Geometry: final body of the model. Coordinates: model frame, mm. A direction names the side the tool comes from. Round coordinates to 2 decimals unless told otherwise and drop trailing zeros. Loops run counter-clockwise (first coordinate to the right, second up) from the corner with the lowest first, then second, coordinate; pieces in that order, holes last. Notation, with made-up numbers: (74, 71.5) - (121, 71.5) arc R25 cw to (121, 108.5) - close; hole circle Ø11 at (17, 57). An arc over 180 degrees is marked (long way). Write item = value, one per line. Start each with the question number.
Item 1: Access query for faces 1 (the flat face through (-11, 33, -6.4)), 2 (the flat face through (-14.8, 74.2, -5.1)), 3 (the flat face through (-19.7, 74, -18)), 4 (the flat face through (-35, 74, -23.025)). Directions: +Z, -Z, +X, -X, +Y, -Y. A direction counts if a zero-diameter tool reaches every point of the face in a straight line with its end or side. Return the directions, or none.
Item 2: Section B-B (x = -32.7). Return loops of the section in (y, z) (3 decimals), plus the area to 3 significant figures.
Item 3: Section C-C (y = 71.5). Return loops of the section in (x, z) (3 decimals), plus the area to 3 significant figures.
Item 4: Draft query along Y for faces 5 (the flat face through (-45.7, 74, -18)), 6 (the cylindrical face through (-53.24, 50.96, 1.48)), 7 (the flat face through (-30, 85.4, -2)). Return one class per face: pulls with the +Y half, pulls with the -Y half, needs draft (parallel to the pull), parting line crosses it, or undercut.
Item 5: Line query: line 1 (Y direction, x = -12.7, z = 0.9); line 2 (Z direction, x = -37, y = 67) (3 decimals); line 3 (Y direction, x = -32.7, z = -25.2). Output: solid intervals per line, ascending. Write a range as from..to.
Item 6: Section D-D (y = 32.7). Return loops of the section in (x, z).
Item 7: First-contact query: pin 1 (1.2 mm diameter, centred on x = -55.5, y = 33, fed in from -Z); pin 2 (2 mm diameter, centred on x = -56, z = -7.5, fed in from +Y); pin 3 (6 mm diameter, centred on y = 74, z = -13.5, fed in from -X); pin 4 (4 mm diameter, centred on x = -24.5, z = -16.5, fed in from +Y). Flat tips, straight axial feed; report the tip coordinate or a pass-through.
Item 8: Section A-A (y = 12). Return loops of the section in (x, z), plus the area to 3 significant figures.
from build123d import *

# Parameters (mm, degrees)
SKETCH_1_W             = 65.4
SKETCH_1_H             = 85.4
SKETCH_1_R             = 2.5
EXTRUDE_632_DEPTH      = 3
SKETCH_2_W             = 26
SKETCH_2_H             = 22
EXTRUDE_871_DEPTH      = 26
SKETCH_3_W             = 20.05
SKETCH_3_H             = 20.05
CUT_EXTRUDE_1082_DEPTH = 95.724442463
SKETCH_8_R             = 5.872551453
EXTRUDE_1_DEPTH        = 14.4
SKETCH_4_R             = 2
EXTRUDE_3_DEPTH        = 14.4
SKETCH_12_R            = 5
EXTRUDE_5_DEPTH        = 21
SKETCH_13_R            = 2
CUT_EXTRUDE_1_DEPTH    = 6.6
SKETCH_14_R            = 2
CUT_EXTRUDE_3_DEPTH    = 8
CHAMFER_1_SIZE         = 10
CHAMFER_2_SIZE         = 10
SKETCH_15_R            = 2
CUT_EXTRUDE_4_DEPTH    = 8


with BuildPart() as part:
    # Эскиз1 → Extrude 632 (new body)
    with BuildSketch(Plane.XY):
        with Locations((-32.7, 42.7)):
            Rectangle(SKETCH_1_W, SKETCH_1_H)
        with Locations((-52.7, 53.4)):
            Circle(SKETCH_1_R, mode=Mode.SUBTRACT)
        with Locations(Location((-12.7, 53.4, 0), (0, 0, 180))):
            Circle(SKETCH_1_R, mode=Mode.SUBTRACT)
        with Locations((-12.7, 12)):
            Circle(SKETCH_1_R, mode=Mode.SUBTRACT)
        with Locations(Location((-52.7, 12, 0), (0, 0, 180))):
            Circle(SKETCH_1_R, mode=Mode.SUBTRACT)
    extrude(amount=EXTRUDE_632_DEPTH)

    # Эскиз2 → Extrude 871 (add)
    with BuildSketch(Plane(origin=(0, 0, 0), x_dir=(-1, 0, 0), z_dir=(0, 0, -1))):
        with Locations((32.7, 74.4)):
            Rectangle(SKETCH_2_W, SKETCH_2_H)
    extrude(amount=EXTRUDE_871_DEPTH)

    # Эскиз3 → Cut-Extrude 1082 (cut, through all)
    with BuildSketch(Plane.XZ.offset(-63.4)):
        with Locations((-32.7, -13)):
            Rectangle(SKETCH_3_W, SKETCH_3_H)
    extrude(amount=-CUT_EXTRUDE_1082_DEPTH, mode=Mode.SUBTRACT)

    # Эскиз8 → Бобышка-Вытянуть1 (add)
    with BuildSketch(Plane(origin=(0, 0, 0), x_dir=(-1, 0, 0), z_dir=(0, 0, -1))):
        with Locations(Location((10.7, 32.7, 0), (0, 0, 180))):
            Circle(SKETCH_8_R)
    extrude(amount=EXTRUDE_1_DEPTH)

    # Эскиз4 → Бобышка-Вытянуть3 (add)
    with BuildSketch(Plane(origin=(0, 0, 0), x_dir=(-1, 0, 0), z_dir=(0, 0, -1))):
        with Locations(Location((52.7, 32.7, 0), (0, 0, 180))):
            Circle(SKETCH_4_R)
    extrude(amount=EXTRUDE_3_DEPTH)

    # Эскиз12 → Бобышка-Вытянуть5 (add)
    with BuildSketch(Plane(origin=(0, 0, 0), x_dir=(-1, 0, 0), z_dir=(0, 0, -1))):
        with Locations(Location((54.7, 32.7, 0), (0, 0, 180))):
            Circle(SKETCH_12_R)
    extrude(amount=EXTRUDE_5_DEPTH)

    # Эскиз13 → Вырез-Вытянуть1 (cut)
    with BuildSketch(Plane(origin=(0, 0, -21), x_dir=(-1, 0, 0), z_dir=(0, 0, -1))):
        with Locations((54.7, 32.7)):
            Circle(SKETCH_13_R)
    extrude(amount=-CUT_EXTRUDE_1_DEPTH, mode=Mode.SUBTRACT)

    # Эскиз14 → Вырез-Вытянуть3 (cut)
    with BuildSketch(Plane(origin=(0, 0, -14.4), x_dir=(-1, 0, 0), z_dir=(0, 0, -1))):
        with Locations((10.7, 32.7)):
            Circle(SKETCH_14_R)
    extrude(amount=-CUT_EXTRUDE_3_DEPTH, mode=Mode.SUBTRACT)

    # Фаска1
    chamfer_1_edges = [part.edges().sort_by_distance(p)[0] for p in [
        (-45.7, 74.4, 0),
    ]]
    chamfer(chamfer_1_edges, length=CHAMFER_1_SIZE)

    # Фаска2
    chamfer_2_edges = [part.edges().sort_by_distance(p)[0] for p in [
        (-19.7, 74.4, 0),
    ]]
    chamfer(chamfer_2_edges, length=CHAMFER_2_SIZE)

    # Эскиз15 → Вырез-Вытянуть4 (cut)
    with BuildSketch(Plane(origin=(0, 0, -26), x_dir=(-1, 0, 0), z_dir=(0, 0, -1))):
        with Locations((32.7, 74.4)):
            Circle(SKETCH_15_R)
    extrude(amount=-CUT_EXTRUDE_4_DEPTH, mode=Mode.SUBTRACT)


solid = part.part
Taken from the geometry:
q1.face_1 = -Z
q1.face_2 = -Z, +X, +Y
q1.face_3 = -Z, +X, +Y, -Y
q1.face_4 = +Y, -Y
q2.outline = (0, 0) - (63.4, 0) - (63.4, -2.975) - (85.4, -2.975) - (85.4, 3) - (0, 3) - close; (63.4, -26) - (72.4, -26) - (72.4, -23.025) - (63.4, -23.025) - close; (76.4, -26) - (85.4, -26) - (85.4, -23.025) - (76.4, -23.025) - close
q2.area = 375 mm^2
q3.outline = (-65.4, 0) - (-55.7, 0) - (-45.7, -10) - (-45.7, -26) - (-19.7, -26) - (-19.7, -10) - (-9.7, 0) - (0, 0) - (0, 3) - (-65.4, 3) - close; hole (-42.725, -23.025) - (-22.675, -23.025) - (-22.675, -2.975) - (-42.725, -2.975) - close
q3.area = 570 mm^2
q4.face_5 = needs draft
q4.face_6 = undercut
q4.face_7 = pulls with the +Y half
q5.line_1 = 0..9.5, 14.5..50.9, 55.9..85.4
q5.line_2 = -26..-23.025, -2.975..3
q5.line_3 = 63.4..72.4, 76.4..85.4
q6.outline = (-65.4, 0) - (-59.7, 0) - (-59.7, -21) - (-56.7, -21) - (-56.7, -14.4) - (-52.7, -14.4) - (-52.7, -21) - (-49.7, -21) - (-49.7, 0) - (-16.57, 0) - (-16.57, -14.4) - (-12.7, -14.4) - (-12.7, -6.4) - (-8.7, -6.4) - (-8.7, -14.4) - (-4.83, -14.4) - (-4.83, 0) - (0, 0) - (0, 3) - (-65.4, 3) - close
q7.pin_1 = -14.4
q7.pin_2 = 37.69
q7.pin_3 = -45.7
q7.pin_4 = 85.4
q8.outline = (-65.4, 0) - (-55.2, 0) - (-55.2, 3) - (-65.4, 3) - close; (-50.2, 0) - (-15.2, 0) - (-15.2, 3) - (-50.2, 3) - close; (-10.2, 0) - (0, 0) - (0, 3) - (-10.2, 3) - close
q8.area = 166 mm^2
